Geometry: final body of the model. Coordinates: model frame, mm. A direction names the side the tool comes from. Round coordinates to 2 decimals unless told otherwise and drop trailing zeros. Loops run counter-clockwise (first coordinate to the right, second up) from the corner with the lowest first, then second, coordinate; pieces in that order, holes last. Notation, with made-up numbers: (8.25, -18.75) - (59.25, -18.75) arc R23 cw to (59.25, 3.25) - close; hole circle Ø1 at (-3, -19.5). An arc over 180 degrees is marked (long way). Use CSV: the item, a comma, the result in double quotes.
from build123d import *

# Parameters (mm, degrees)
SKETCH1_R           = 15
SKETCH1_R_2         = 2.5
BOSS_EXTRUDE1_DEPTH = 5
BOSS_EXTRUDE2_START = -5
SKETCH2_R           = 17
SKETCH2_R_2         = 15
BOSS_EXTRUDE2_DEPTH = 5
SKETCH3_R           = 18
CUT_EXTRUDE1_DEPTH  = 5
SKETCH4_R           = 18.354217927
CUT_EXTRUDE2_DEPTH  = 5


with BuildPart() as part:
    # Sketch1 → Boss-Extrude1 (new body)
    with BuildSketch(Plane(origin=(0, 0, 0), x_dir=(1, 0, 0), z_dir=(0, 1, 0))):
        with Locations(Location((0, 0, 0), (0, 0, 270))):
            Circle(SKETCH1_R)
        with Locations(Location((0, 0, 0), (0, 0, 270))):
            Circle(SKETCH1_R_2, mode=Mode.SUBTRACT)
    extrude(amount=BOSS_EXTRUDE1_DEPTH)

    # Sketch2 → Boss-Extrude2 (add)
    with BuildSketch(Plane(origin=(0, 5, 0), x_dir=(1, 0, 0), z_dir=(0, 1, 0)).offset(BOSS_EXTRUDE2_START)):
        with Locations(Location((0, 0, 0), (0, 0, 270))):
            Circle(SKETCH2_R)
        Circle(SKETCH2_R_2, mode=Mode.SUBTRACT)
    extrude(amount=BOSS_EXTRUDE2_DEPTH)

    # Sketch3 → Cut-Extrude1 (cut)
    with BuildSketch(Plane(origin=(0, 5, 0), x_dir=(1, 0, 0), z_dir=(0, 1, 0))):
        Circle(SKETCH3_R)
        Polygon((0.800081407, 17), (-0.800081407, 17), (-2.565946388, 12.667519465), (-3.338765682, 12.460443159), (-4.111584976, 12.253366853), (-7.807109176, 15.122472568), (-9.192890824, 14.322391161), (-8.555934489, 9.687420466), (-9.121677477, 9.121677477), (-9.687420466, 8.555934489), (-14.322391161, 9.192890824), (-15.122472568, 7.807109176), (-12.253366853, 4.111584976), (-12.460443159, 3.338765682), (-12.667519465, 2.565946388), (-17, 0.800081407), (-17, -0.800081407), (-12.667519465, -2.565946388), (-12.460443159, -3.338765682), (-12.253366853, -4.111584976), (-15.122472568, -7.807109176), (-14.322391161, -9.192890824), (-9.687420466, -8.555934489), (-9.121677477, -9.121677477), (-8.555934489, -9.687420466), (-9.192890824, -14.322391161), (-7.807109176, -15.122472568), (-4.111584976, -12.253366853), (-3.338765682, -12.460443159), (-2.565946388, -12.667519465), (-0.800081407, -17), (0.800081407, -17), (2.565946388, -12.667519465), (3.338765682, -12.460443159), (4.111584976, -12.253366853), (7.807109176, -15.122472568), (9.192890824, -14.322391161), (8.555934489, -9.687420466), (9.121677477, -9.121677477), (9.687420466, -8.555934489), (14.322391161, -9.192890824), (15.122472568, -7.807109176), (12.253366853, -4.111584976), (12.460443159, -3.338765682), (12.667519465, -2.565946388), (17, -0.800081407), (17, 0.800081407), (12.667519465, 2.565946388), (12.460443159, 3.338765682), (12.253366853, 4.111584976), (15.122472568, 7.807109176), (14.322391161, 9.192890824), (9.687420466, 8.555934489), (9.121677477, 9.121677477), (8.555934489, 9.687420466), (9.192890824, 14.322391161), (7.807109176, 15.122472568), (4.111584976, 12.253366853), (3.338765682, 12.460443159), (2.565946388, 12.667519465), align=None, mode=Mode.SUBTRACT)
    extrude(amount=-CUT_EXTRUDE1_DEPTH, mode=Mode.SUBTRACT)

    # Sketch4 → Cut-Extrude2 (cut)
    with BuildSketch(Plane(origin=(0, 5, 0), x_dir=(1, 0, 0), z_dir=(0, 1, 0))):
        Circle(SKETCH4_R)
        with BuildLine():
            Line((2.492089445, 12.583781755), (4.133678109, 12.143919398))
            Line((4.133678109, 12.143919398), (7.801525521, 14.991537598))
            ThreePointArc((7.801525521, 14.991537598), (8.45, 14.635829324), (9.082289641, 14.252088088))
            Line((9.082289641, 14.252088088), (8.450103646, 9.651829953))
            Line((8.450103646, 9.651829953), (9.651829953, 8.450103646))
            Line((9.651829953, 8.450103646), (14.252088088, 9.082289641))
            ThreePointArc((14.252088088, 9.082289641), (14.635829324, 8.45), (14.991537598, 7.801525521))
            Line((14.991537598, 7.801525521), (12.143919398, 4.133678109))
            Line((12.143919398, 4.133678109), (12.583781755, 2.492089445))
            Line((12.583781755, 2.492089445), (16.883815162, 0.739449509))
            ThreePointArc((16.883815162, 0.739449509), (16.9, 0), (16.883815162, -0.739449509))
            Line((16.883815162, -0.739449509), (12.583781755, -2.492089445))
            Line((12.583781755, -2.492089445), (12.143919398, -4.133678109))
            Line((12.143919398, -4.133678109), (14.991537598, -7.801525521))
            ThreePointArc((14.991537598, -7.801525521), (14.635829324, -8.45), (14.252088088, -9.082289641))
            Line((14.252088088, -9.082289641), (9.651829953, -8.450103646))
            Line((9.651829953, -8.450103646), (8.450103646, -9.651829953))
            Line((8.450103646, -9.651829953), (9.082289641, -14.252088088))
            ThreePointArc((9.082289641, -14.252088088), (8.45, -14.635829324), (7.801525521, -14.991537598))
            Line((7.801525521, -14.991537598), (4.133678109, -12.143919398))
            Line((4.133678109, -12.143919398), (2.492089445, -12.583781755))
            Line((2.492089445, -12.583781755), (0.739449509, -16.883815162))
            ThreePointArc((0.739449509, -16.883815162), (0, -16.9), (-0.739449509, -16.883815162))
            Line((-0.739449509, -16.883815162), (-2.492089445, -12.583781755))
            Line((-2.492089445, -12.583781755), (-4.133678109, -12.143919398))
            Line((-4.133678109, -12.143919398), (-7.801525521, -14.991537598))
            ThreePointArc((-7.801525521, -14.991537598), (-8.45, -14.635829324), (-9.082289641, -14.252088088))
            Line((-9.082289641, -14.252088088), (-8.450103646, -9.651829953))
            Line((-8.450103646, -9.651829953), (-9.651829953, -8.450103646))
            Line((-9.651829953, -8.450103646), (-14.252088088, -9.082289641))
            ThreePointArc((-14.252088088, -9.082289641), (-14.635829324, -8.45), (-14.991537598, -7.801525521))
            Line((-14.991537598, -7.801525521), (-12.143919398, -4.133678109))
            Line((-12.143919398, -4.133678109), (-12.583781755, -2.492089445))
            Line((-12.583781755, -2.492089445), (-16.883815162, -0.739449509))
            ThreePointArc((-16.883815162, -0.739449509), (-16.9, 0), (-16.883815162, 0.739449509))
            Line((-16.883815162, 0.739449509), (-12.583781755, 2.492089445))
            Line((-12.583781755, 2.492089445), (-12.143919398, 4.133678109))
            Line((-12.143919398, 4.133678109), (-14.991537598, 7.801525521))
            ThreePointArc((-14.991537598, 7.801525521), (-14.635829324, 8.45), (-14.252088088, 9.082289641))
            Line((-14.252088088, 9.082289641), (-9.651829953, 8.450103646))
            Line((-9.651829953, 8.450103646), (-8.450103646, 9.651829953))
            Line((-8.450103646, 9.651829953), (-9.082289641, 14.252088088))
            ThreePointArc((-9.082289641, 14.252088088), (-8.45, 14.635829324), (-7.801525521, 14.991537598))
            Line((-7.801525521, 14.991537598), (-4.133678109, 12.143919398))
            Line((-4.133678109, 12.143919398), (-2.492089445, 12.583781755))
            Line((-2.492089445, 12.583781755), (-0.739449509, 16.883815162))
            ThreePointArc((-0.739449509, 16.883815162), (0, 16.9), (0.739449509, 16.883815162))
            Line((0.739449509, 16.883815162), (2.492089445, 12.583781755))
        make_face(mode=Mode.SUBTRACT)
    extrude(amount=-CUT_EXTRUDE2_DEPTH, mode=Mode.SUBTRACT)


solid = part.part
Item 1: Mould query, pull axis Z, two halves, no side actions, for faces 4 (the flat face through (-5.993, 2.535, -13.588)), 5 (the flat face through (-4, 5, 0)), 6 (the flat face through (9, 2.5, -9.1)), 7 (the cylindrical face through (-8.44, 2.54, 14.64)). Classes: released by +Z, released by -Z, zero draft, split by the parting line, or undercut.
Final values:
face 4,"released by -Z"
face 5,"zero draft"
face 6,"undercut"
face 7,"released by +Z"
Item 2: Reachability of faces 1 (the flat face through (3.301, 2.535, -12.367)), 2 (the flat face through (8.76, 2.54, 11.92)), 3 (the flat face through (5.993, 2.535, 13.588)) from +Z, -Z, +X, -X, +Y, -Y: full face, straight path, thin tool, end or side. Return the list, or none.
Final values:
face 1,"-Z, +Y, -Y"
face 2,"+X, +Y, -Y"
face 3,"+Z, +Y, -Y"
Item 3: Section C-C on x = 11.5. Return the cut outline in (y, z).
Final values:
outline,"(0, -8.7) - (5, -8.7) - (5, 8.7) - (0, 8.7) - close"
Item 4: Section A-A on x = 0. Return the cut outline in (y, z).
Final values:
outline,"(0, -16.9) - (5, -16.9) - (5, -2.5) - (0, -2.5) - close; (0, 2.5) - (5, 2.5) - (5, 16.9) - (0, 16.9) - close"
Item 5: Section B-B on z = 0. Return the cut outline in (x, y), plus the area to 3 significant figures.
Final values:
outline,"(-16.9, 0) - (-2.5, 0) - (-2.5, 5) - (-16.9, 5) - close; (2.5, 0) - (16.9, 0) - (16.9, 5) - (2.5, 5) - close"
area,"144 mm²"
Item 6: Pin query (flat end, axial travel): P1, Ø1.5, axis at y = 1, z = 4.5, coming from the -X side; P2, Ø1.5, axis at y = 3, z = 5, coming from the -X side; P3, Ø4, axis at x = 4.5, z = 7, coming from the -Y side. Return the tip coordinate at first contact, or that it passes through.
Final values:
P1,"stops at x = -13.01"
P2,"stops at x = -13.4"
P3,"stops at y = 0"
Item 7: Material intervals for line 1 (X direction, y = 1.3, z = 0); line 2 (Z direction, x = 1, y = 0.2); line 3 (Z direction, x = 12, y = 1.35), sorted ascending.
Final values:
line 1,"x = -16.9 to -2.5, 2.5 to 16.9"
line 2,"z = -16.24 to -2.29, 2.29 to 16.24"
line 3,"z = -8.77 to 8.77"
